Autodesk Inventor part; units mm, degrees
ref_plane "YZ Plane" through (0, 0, 0) normal (1, 0, 0) x (0, 1, 0)
ref_plane "XZ Plane" through (0, 0, 0) normal (0, 1, 0) x (-1, 0, 0)
ref_plane "XY Plane" through (0, 0, 0) normal (0, 0, 1) x (1, 0, 0)
sketch "Sketch1" plane through (0, 0, 0) normal (0, 1, 0) x (-1, 0, 0)
  circle A0 centre (66.0648, 12.7211) radius 2.5
  circle A1 centre (66.0648, 12.7211) radius 2.5
  point P0 (0, 0)
  dimension "d7" = 5
extrude "Extrusion1" add sketch "Sketch1" along normal blind 16
sketch "Sketch2" plane through (-66.0648, 16, 12.7211) normal (0, 1, 0) x (1, 0, 0)
  line L0 (0.8397, 1.4867) -> (-0.9155, 1.4912)
  ellipse E0 centre (0.0567, 0.0303) end of major axis (-0.8862, 1.7941) minor radius 1.9327 (-1.2692, 1.5225) -> (1.3068, 1.516) ccw
  spline S0 degree 2 poles (1.3068, 1.516) (1.0542, 1.4985) (0.8397, 1.4867) knots 0 0 0 1 1 1 weights 1 1.006377 1
  spline S1 degree 2 poles (-0.9155, 1.4912) (-1.084, 1.5039) (-1.2692, 1.5225) knots 0 0 0 1 1 1 weights 1 1.006377 1
  point P0 (66.0648, 12.7211)
  point P1 (-1.3518, 1.4745)
extrude "Extrusion5" cut sketch "Sketch2" against normal blind 9
properties part number "acoplador"
Geometry check sheet. Reference: the model listing, model coordinates, mm. Coordinates: 2 decimals unless noted, no trailing zeros. Order: outer loops, then holes, each group sorted by start corner. A loop starts at its lowest first (then second) coordinate and runs counter-clockwise, first axis right, second up. Notation, with made-up numbers: (75.25, 13.25) - (116.25, 13.25) arc R10 cw to (116.25, 27.25) - close; hole circle Ø2 at (55.25, 68). An arc over 180 degrees is marked (long way). Answer in a Markdown table with one row per item. Add a question column.
1. Section check A-A (y = 1.5). Enter the section's corners in (x, z), plus the area to 3 significant figures.
2. Material ranges on L1, parallel to Z at x = -66, y = 8.5; L2, parallel to Y at x = -66.1, z = 11.8; L3, parallel to Z at x = -67.7, y = 8, recorded low to high. Write a range as [from, to].
3. Draft check along X on faces 1 (the face through (-68.45, 7.89, 11.97)), 2 (the face through (-66, 7, 13)), 3 (the face through (-66, 16, 11)). Enter one of: +X half, -X half, draft (parallel to the pull), parting line (faces both ways), or undercut.
Data:
| question | item | result |
|---|---|---|
| 1 | outline | circle Ø5 at (-66.06, 12.72) |
| 1 | area | 19.6 mm² |
| 2 | L1 | z = [10.22, 11.23], [14.68, 15.22] |
| 2 | L2 | y = [0, 7] |
| 2 | L3 | z = [10.83, 11.66], [13.63, 14.61] |
| 3 | face 1 | parting line |
| 3 | face 2 | undercut |
| 3 | face 3 | draft |
